Geometry: final body of the model. Coordinates: model frame, mm. A direction names the side the tool comes from. Coordinates: 2 decimals unless noted, no trailing zeros. Write each loop counter-clockwise with the first axis right and the second up, starting at its lowest first coordinate (ties: lowest second). Pieces come first, ordered by that corner, then holes. Notation, with made-up numbers: (25, 0.5) -> (48, 0.5) arc R24 ccw to (48, 30.5) -> close; hole circle Ø9 at (-15, 72.5). An arc over 180 degrees is marked (long way). Answer as a JSON object with one key per item and string values. Group by question number.
```python
from build123d import *

# Parameters (mm, degrees)
EXTRUDE_1_DEPTH = 25
SHELL_1_T       = -2.2


with BuildPart() as part:
    # Эскиз1 → Бобышка-Вытянуть1 (new body)
    with BuildSketch(Plane.XY):
        with BuildLine():
            Line((-503.628105098, 213.614457831), (321.371894902, 213.614457831))
            ThreePointArc((321.371894902, 213.614457831), (356.727233962, 198.969796891), (371.371894902, 163.614457831))
            Line((371.371894902, 163.614457831), (371.371894902, 88.614457831))
            Line((371.371894902, 88.614457831), (396.371894902, 88.614457831))
            Line((396.371894902, 88.614457831), (396.371894902, 163.614457831))
            ThreePointArc((396.371894902, 163.614457831), (374.404903491, 216.64746642), (321.371894902, 238.614457831))
            Line((321.371894902, 238.614457831), (-503.628105098, 238.614457831))
            Line((-503.628105098, 238.614457831), (-503.628105098, 213.614457831))
        make_face()
    extrude(amount=EXTRUDE_1_DEPTH)

    # Оболочка1
    shell_1_openings = [part.faces().sort_by_distance(p)[0] for p in [
        (383.871894902, 88.614457831, 12.5),
        (-503.628105098, 226.114457831, 12.5),
    ]]
    offset(amount=SHELL_1_T, openings=shell_1_openings, kind=Kind.INTERSECTION)


solid = part.part
```
Item 1: Section A-A on z = 15.5. Output: boundary loops of the cut face in (x, y), then the cut area to 3 significant figures.
Item 2: Set-up query: faces 4 (the flat face through (10, 218, 2.2)), 5 (the flat face through (-97, 215.814, 12)), 6 (the flat face through (371.372, 127, 12)), 7 (the flat face through (373.572, 127, 12)). Return all of +Z, -Z, +X, -X, +Y, -Y with unobstructed straight access to the full face (end or side cutting, diameter ignored); none if empty.
Item 3: Contact query for flat-ended pins moving along their axis: pin 1 (8 mm diameter, centred on x = -216, z = 8, fed in from -Y); pin 2 (2 mm diameter, centred on y = 158, z = 13, fed in from -X); pin 3 (12 mm diameter, centred on y = 184.5, z = 16, fed in from +X). Output: stop coordinate, or through.
Item 4: Section B-B on y = 100.5. Output: boundary loops of the cut face in (x, z), then the cut area to 3 significant figures.
Item 5: Ray query, L1, parallel to Y at x = -33.5, z = 14.25; L2, parallel to X at y = 144, z = 21.75; L3, parallel to X at y = 178.5, z = 9.75. Return the intervals inside material, ascending. Write a range as [from, to].
Item 6: Section D-D on y = 228. Output: boundary loops of the cut face in (x, z).
Item 7: Section C-C on x = -34. Output: boundary loops of the cut face in (y, z), then the cut area to 3 significant figures.
Item 8: Mould query, pull axis X, two halves, no side actions, for faces 1 (the flat face through (394.172, 126, 12)), 2 (the flat face through (-85, 236.414, 12)), 3 (the cylindrical face through (356.336, 199.356, 12.325)). Classes: +X half, -X half, draft (parallel to the pull), parting line (faces both ways), or undercut.
Answer sheet:
{
 "1": {"outline": "(-503.63, 213.61) -> (321.37, 213.61) arc R50 cw to (371.37, 163.61) -> (371.37, 88.61) -> (373.57, 88.61) -> (373.57, 163.61) arc R52.2 ccw to (321.37, 215.81) -> (-503.63, 215.81) -> close; (-503.63, 236.41) -> (321.37, 236.41) arc R72.8 cw to (394.17, 163.61) -> (394.17, 88.61) -> (396.37, 88.61) -> (396.37, 163.61) arc R75 ccw to (321.37, 238.61) -> (-503.63, 238.61) -> close", "area": "4,390 mm^2"},
 "2": {"face 4": "none", "face 5": "-X", "face 6": "+Z, -Z, -X, -Y", "face 7": "-Y"},
 "3": {"pin 1": "stops at y = 213.61", "pin 2": "stops at x = 371.37", "pin 3": "stops at x = 394.88"},
 "4": {"outline": "(371.37, 0) -> (396.37, 0) -> (396.37, 25) -> (371.37, 25) -> close; hole (373.57, 2.2) -> (394.17, 2.2) -> (394.17, 22.8) -> (373.57, 22.8) -> close", "area": "201 mm^2"},
 "5": {"L1": "y = [213.61, 215.81], [236.41, 238.61]", "L2": "x = [371.37, 373.57], [394.17, 396.37]", "L3": "x = [369.1, 371.4], [392.63, 394.88]"},
 "6": {"outline": "(-503.63, 0) -> (359.84, 0) -> (359.84, 25) -> (-503.63, 25) -> (-503.63, 22.8) -> (355.35, 22.8) -> (355.35, 2.2) -> (-503.63, 2.2) -> close"},
 "7": {"outline": "(213.61, 0) -> (238.61, 0) -> (238.61, 25) -> (213.61, 25) -> close; hole (215.81, 2.2) -> (236.41, 2.2) -> (236.41, 22.8) -> (215.81, 22.8) -> close", "area": "201 mm^2"},
 "8": {"face 1": "undercut", "face 2": "draft", "face 3": "-X half"}
}
